Check sheet for the modelled part. Datum: model origin and axes. Units: mm. A direction names the side the tool comes from. Round coordinates to 2 decimals unless told otherwise and drop trailing zeros. Loops run counter-clockwise (first coordinate to the right, second up) from the corner with the lowest first, then second, coordinate; pieces in that order, holes last. Notation, with made-up numbers: (49, -35.5) -> (90, -35.5) arc R11 cw to (90, -15.5) -> close; hole circle Ø11 at (7.5, 72.25). An arc over 180 degrees is marked (long way). Return JSON: item names as keys, results as strings.
from build123d import *

# Parameters (mm, degrees)
BOSS_EXTRUDE1_DEPTH = 5
SKETCH3_R           = 2.5
SKETCH3_W           = 20
SKETCH3_H           = 40.5
CUT_EXTRUDE3_DEPTH  = 189.745860882
FILLET1_R           = 5
FILLET2_R           = 5
FILLET3_R           = 5
FILLET4_R           = 5
FILLET5_R           = 5
FILLET6_R           = 5
SKETCH4_W           = 5
SKETCH4_H           = 7
CUT_EXTRUDE6_DEPTH  = 189.745860882


with BuildPart() as part:
    # Sketch1 → Boss-Extrude1 (new body)
    with BuildSketch(Plane.XY):
        Polygon((0, 40), (30, 10), (70, 10), (100, 40), (100, 160), (0, 160), align=None)
    extrude(amount=BOSS_EXTRUDE1_DEPTH)

    # Sketch3 → Cut-Extrude3 (cut, through all)
    with BuildSketch(Plane.XY.offset(5)):
        with Locations((50, 20)):
            Circle(SKETCH3_R)
        with Locations((85, 63)):
            Circle(SKETCH3_R)
        with Locations((15, 63)):
            Circle(SKETCH3_R)
        with Locations((60, 98.25)):
            Rectangle(SKETCH3_W, SKETCH3_H)
        with BuildLine():
            Line((35, 49.5), (65, 49.5))
            ThreePointArc((65, 49.5), (73, 41.5), (65, 33.5))
            Line((65, 33.5), (35, 33.5))
            ThreePointArc((35, 33.5), (27, 41.5), (35, 49.5))
        make_face()
    extrude(amount=-CUT_EXTRUDE3_DEPTH, mode=Mode.SUBTRACT)

    # Fillet1
    fillet1_edges = [part.edges().sort_by_distance(p)[0] for p in [
        (0, 40, 2.5),
    ]]
    fillet(fillet1_edges, radius=FILLET1_R)

    # Fillet2
    fillet2_edges = [part.edges().sort_by_distance(p)[0] for p in [
        (100, 40, 2.5),
    ]]
    fillet(fillet2_edges, radius=FILLET2_R)

    # Fillet3
    fillet3_edges = [part.edges().sort_by_distance(p)[0] for p in [
        (70, 10, 2.5),
    ]]
    fillet(fillet3_edges, radius=FILLET3_R)

    # Fillet4
    fillet4_edges = [part.edges().sort_by_distance(p)[0] for p in [
        (30, 10, 2.5),
    ]]
    fillet(fillet4_edges, radius=FILLET4_R)

    # Fillet5
    fillet5_edges = [part.edges().sort_by_distance(p)[0] for p in [
        (100, 160, 2.5),
    ]]
    fillet(fillet5_edges, radius=FILLET5_R)

    # Fillet6
    fillet6_edges = [part.edges().sort_by_distance(p)[0] for p in [
        (0, 160, 2.5),
    ]]
    fillet(fillet6_edges, radius=FILLET6_R)

    # Sketch4 → Cut-Extrude6 (cut, through all)
    with BuildSketch(Plane.XY.offset(5)):
        with Locations((7.5, 41.5)):
            Rectangle(SKETCH4_W, SKETCH4_H)
        with Locations((92.5, 41.5)):
            Rectangle(SKETCH4_W, SKETCH4_H)
    extrude(amount=-CUT_EXTRUDE6_DEPTH, mode=Mode.SUBTRACT)


solid = part.part
Q1. Material ranges on line 1 (Y direction, x = 61, z = 3.35); line 2 (Y direction, x = 45, z = 0.25); line 3 (X direction, y = 102, z = 0.9), recorded low to high.
Results list:
{"line 1": "10 to 33.5, 49.5 to 78, 118.5 to 160", "line 2": "10 to 33.5, 49.5 to 160", "line 3": "0 to 50, 70 to 100"}
Q2. Section check D-D (z = 3.05). Count the separate pieces of the cut face and the enclosed holes in it, then the cut area to 3 significant figures.
Results list:
{"separate pieces": "1", "enclosed holes": "7", "area": "12,500 mm^2"}
Q3. Tool access check on faces 1 (the cylindrical face through (2, 159, 3)), 2 (the flat face through (50, 49.5, 3)). Record the directions out of +Z, -Z, +X, -X, +Y, -Y that give a thin tool (end or side, any length) a straight path to the whole face; none if there is none.
Results list:
{"face 1": "+Z, -Z, -X, +Y", "face 2": "+Z, -Z"}
Q4. Go/stop test with flat-tipped pins: pin 1 (12 mm diameter, centred on x = 63, y = 129, fed in from -Z); pin 2 (2.5 mm diameter, centred on y = 40.5, z = 3, fed in from +X); pin 3 (4.5 mm diameter, centred on x = 50, y = 20, fed in from -Z); pin 4 (1.5 mm diameter, centred on x = 76, z = 3.5, fed in from -Y). Record where each tip stops, or that it passes through.
Results list:
{"pin 1": "z = 0", "pin 2": "x = 99.99", "pin 3": "through", "pin 4": "y = 15.25"}
Q5. Draft check along X on faces 3 (the cylindrical face through (0.39, 40.13, 2.54)), 4 (the flat face through (51, 160, 2)), 5 (the flat face through (7, 38, 3)). Enter one of: released by +X, released by -X, zero draft, split by the parting line, or undercut.
Results list:
{"face 3": "released by -X", "face 4": "zero draft", "face 5": "undercut"}
Q6. Section check C-C (y = 63). Record the boundary of the cut face in (x, z), then the cut area to 3 significant figures.
Results list:
{"outline": "(0, 0) -> (12.5, 0) -> (12.5, 5) -> (0, 5) -> close; (17.5, 0) -> (82.5, 0) -> (82.5, 5) -> (17.5, 5) -> close; (87.5, 0) -> (100, 0) -> (100, 5) -> (87.5, 5) -> close", "area": "450 mm^2"}
Q7. Section check A-A (x = 36.5). Record the boundary of the cut face in (y, z), then the cut area to 3 significant figures.
Results list:
{"outline": "(10, 0) -> (33.5, 0) -> (33.5, 5) -> (10, 5) -> close; (49.5, 0) -> (160, 0) -> (160, 5) -> (49.5, 5) -> close", "area": "670 mm^2"}
Q8. Section check B-B (y = 20). Record the boundary of the cut face in (x, z).
Results list:
{"outline": "(20, 0) -> (47.5, 0) -> (47.5, 5) -> (20, 5) -> close; (52.5, 0) -> (80, 0) -> (80, 5) -> (52.5, 5) -> close"}
